Part print with two shaded views. Sizes in mm from the minimum x, y, z corner. A direction names the side the tool comes from. Give positions to 0.01 mm unless a question says otherwise; leave off trailing zeros. Write each loop counter-clockwise with the first axis right and the second up, starting at its lowest first coordinate (ties: lowest second). Pieces come first, ordered by that corner, then holes.
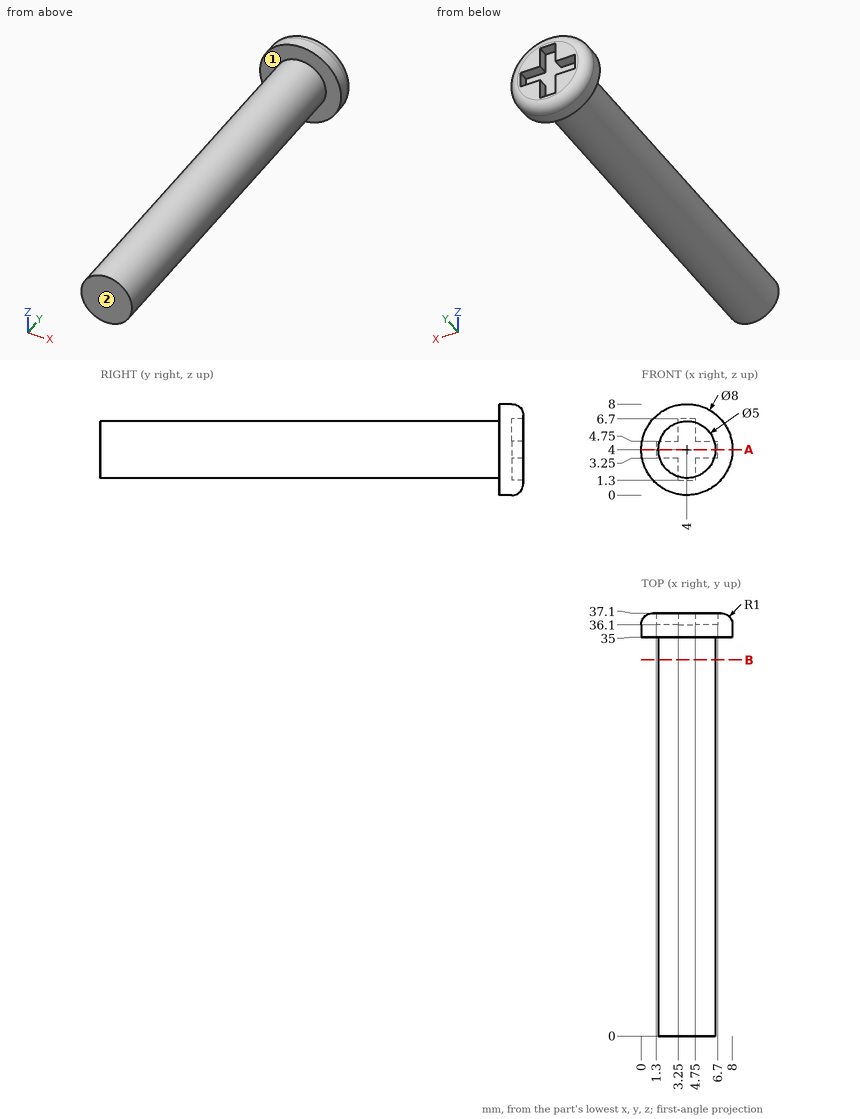
1) Saw through at A-A (z = 4). Write the cut outline in (x, y), and give its area (3 significant figures).
Check result:
outline: (0, 35) - (1.5, 35) - (1.5, 0) - (6.5, 0) - (6.5, 35) - (8, 35) - (8, 36.1) arc R1 ccw to (7, 37.1) - (6.7, 37.1) - (6.7, 36.1) - (1.3, 36.1) - (1.3, 37.1) - (1, 37.1) arc R1 ccw to (0, 36.1) - close
area: 186 mm2
2) Flat gauge pins, fed straight in: P1, Ø0.5, axis at y = 36.5, z = 2.5, coming from the +X side; P2, Ø1.5, axis at y = 22.5, z = 4.5, coming from the -X side; P3, Ø0.8, axis at x = 6, y = 36.5, coming from the +Z side. Where does each tip first touch, or does it go through?
Check result:
P1: stops at x = 7.75
P2: stops at x = 1.5
P3: stops at z = 7.62
3) 3-axis set-ups, long thin cutter, end or side, ignore diameter. For the marked faces 1 and 2: which of +Z, -Z, +X, -X, +Y, -Y reach the whole face in a straight line?
Check result:
face 1: -Y
face 2: +Z, -Z, +X, -X, -Y
4) Drill centre lines: L1, parallel to Z at x = 4, y = 21; L2, parallel to Y at x = 6.75, z = 4.5. Where is each one in solid material? Low to high.
Check result:
L1: z = 1.5 to 6.5
L2: y = 35 to 37.1
5) Saw through at B-B (y = 33). Write the cut outline in (x, z), and give its area (3 significant figures).
Check result:
outline: circle Ø5 at (4, 4)
area: 19.6 mm2
